from build123d import *

# Parameters (mm, degrees)
BOSS_EXTRUDE1_DEPTH = 8
SKETCH2_R           = 7.6
CUT_EXTRUDE1_DEPTH  = 26
FILLET1_R           = 1


with BuildPart() as part:
    # Sketch1 → Boss-Extrude1 (new body, symmetric)
    with BuildSketch(Plane.XY):
        with BuildLine():
            Line((8, 4), (-8, 4))
            Line((-8, 4), (-8, -4))
            Line((-8, -4), (-6.049793385, -4))
            ThreePointArc((-6.049793385, -4), (0, -1), (6.049793385, -4))
            Line((6.049793385, -4), (8, -4))
            Line((8, -4), (8, 4))
        make_face()
    extrude(amount=BOSS_EXTRUDE1_DEPTH, both=True)

    # Sketch2 → Cut-Extrude1 (cut)
    with BuildSketch(Plane.ZY.offset(8)):
        with Locations((0, 8.6)):
            Circle(SKETCH2_R)
    extrude(amount=-CUT_EXTRUDE1_DEPTH, mode=Mode.SUBTRACT)

    # Fillet1
    fillet1_edges = [part.edges().sort_by_distance(p)[0] for p in [
        (8, -4, 0),
        (-8, -4, 0),
        (0, 4, -8),
        (0, 4, 8),
    ]]
    fillet(fillet1_edges, radius=FILLET1_R)


solid = part.part
Design review of the part built by this model. Coordinates are the model's own, in mm. Give positions to 0.01 mm unless a question says otherwise; leave off trailing zeros. Order: outer loops, then holes, each group sorted by start corner. A loop starts at its lowest first (then second) coordinate and runs counter-clockwise, first axis right, second up.
1. For pin 1 Ø1 at (x, z) = (4.5, -0.5) entering from -Y; pin 2 Ø2 at (y, z) = (2.5, 3.5) entering from +X; pin 3 Ø2 at (x, z) = (4, 2) entering from +Y, all flat-tipped, find the tip position at first contact; note any pin that passes through.
Solution:
pin 1: stops at y = -2.88
pin 2: stops at x = 8
pin 3: stops at y = 1.62
2. Add section A-A, the plane y = -2.75. State the section outline as (x, z) points.
Solution:
outline: (-8, -8) - (-4.85, -8) - (-4.85, 8) - (-8, 8) - close; (4.85, -8) - (8, -8) - (8, 8) - (4.85, 8) - close
3. Add section C-C, the plane z = 4.5. State the section outline as (x, y) points, then the cut area to 3 significant figures.
Solution:
outline: (-8, -3) arc R1 ccw to (-7, -4) - (-6.05, -4) arc R7.6 cw to (6.05, -4) - (7, -4) arc R1 ccw to (8, -3) - (8, 2.48) - (-8, 2.48) - close
area: 77.8 mm2
4. Add section B-B, the plane x = -1.25. State the section outline as (y, z) points, then the cut area to 3 significant figures.
Solution:
outline: (-1.1, -8) - (3, -8) arc R1 ccw to (4, -7) - (4, -6.05) arc R7.6 cw to (4, 6.05) - (4, 7) arc R1 ccw to (3, 8) - (-1.1, 8) - close
area: 55.9 mm2
5. Mouldability with a two-part tool opening along Z and no side actions: class faces 1 (the flat face through (0, 0, -8)), 2 (the cylindrical face through (0, 1, 0)), 3 (the flat face through (6.5, -4, 0.1)), 4 (the flat face through (0, 0, 8)) as +Z half, -Z half, draft (parallel to the pull), parting line (faces both ways), or undercut.
Solution:
face 1: -Z half
face 2: undercut
face 3: draft
face 4: +Z half
6. To check wall thickness, follow L1, parallel to Z at x = 0, y = 2.75; L2, parallel to X at y = -2, z = 3; L3, parallel to Z at x = -0.75, y = 2.5. State the ranges of each line that lie inside material, in increasing order.
Solution:
L1: z = -8 to -4.85, 4.85 to 8
L2: x = -8 to -3.77, 3.77 to 8
L3: z = -8 to -4.53, 4.53 to 8
